Model file for the job. Use its own axes, mm. A direction names the side the tool comes from. Give positions to 0.01 mm unless a question says otherwise; leave off trailing zeros. Order: outer loops, then holes, each group sorted by start corner. A loop starts at its lowest first (then second) coordinate and runs counter-clockwise, first axis right, second up. Notation, with made-up numbers: (15.25, 45.5) -> (36.25, 45.5) arc R19 ccw to (36.25, 72.5) -> close; hole circle Ø8 at (64.5, -15.5). An arc over 180 degrees is marked (long way). Use CSV: the item, a comma, the result in double quotes. Start each with the question number.
1. Pull direction Y, two halves, no side cores. Call faces 4 (the flat face through (59, 0, 49)), 5 (the flat face through (61, 77, 49)), 6 (the flat face through (0, 79, 50)), 7 (the flat face through (61, 80, 49)): released by +Y, released by -Y, zero draft, split by the parting line, or undercut.
2. Cut at C-C on z = 71.5. List the corners of the cut face in (x, y), then the cut area to 3 significant figures.
3. Cut at D-D on z = 23. List the corners of the cut face in (x, y), then the cut area to 3 significant figures.
4. Drop flat-ended pins along their axis: pin 1 (4 mm diameter, centred on x = 115, z = 23, fed in from -Y); pin 2 (4.5 mm diameter, centred on x = 97.577, y = 59.65, fed in from -Z). Give the stop position or say it passes through.
5. Cut at A-A on x = 5. List the corners of the cut face in (y, z), then the cut area to 3 significant figures.
6. Cut at B-B on y = 20.35. List the corners of the cut face in (x, z), then the cut area to 3 significant figures.
7. 3-axis set-ups, long thin cutter, end or side, ignore diameter. For faces 1 (the cylindrical face through (39.04, 35.67, 1.52)), 2 (the flat face through (61, 41, 97)), 3 (the cylindrical face through (45.586, 19.392, 1.521)): which of +Z, -Z, +X, -X, +Y, -Y reach the whole face in a straight line?
8. Wall check: line 1 (Z direction, x = 59.5, y = 34); line 2 (Y direction, x = 107, z = 15); line 3 (Y direction, x = 40, z = 2.2) (3 decimals). Give the ranges that are in metal, low to high. Write a range as from..to.
Autodesk Inventor part; units mm, degrees
ref_plane "Work Plane1" through (0, 0, 50) normal (0, 0, 1) x (1, 0, 0)
ref_plane "YZ Plane" through (0, 0, 0) normal (1, 0, 0) x (0, 1, 0)
ref_plane "XZ Plane" through (0, 0, 0) normal (0, 1, 0) x (-1, 0, 0)
sketch "Sketch6" plane through (0, 0, 0) normal (0, 0, 1) x (1, 0, 0)
  line L0 (0, 0) -> (120, 0)
  line L1 (120, 0) -> (120, 80)
  line L2 (120, 80) -> (0, 80)
  line L3 (0, 80) -> (0, 0)
  dimension "d18" = 80
  dimension "d19" = 120
extrude "Extrusion4" add sketch "Sketch6" along normal blind 100
sketch "Sketch7" plane through (120, 0, 0) normal (1, 0, 0) x (0, 0, -1)
  line L0 (0, 0) -> (0, 80)
  line L1 (0, 80) -> (-100, 80)
  line L2 (-100, 0) -> (-100, 80)
  line L3 (0, 0) -> (-100, 0)
  line L4 (-97, 3) -> (-3, 3)
  line L5 (-3, 3) -> (-3, 77)
  line L6 (-3, 77) -> (-97, 77)
  line L7 (-97, 77) -> (-97, 3)
  point P0 (0, 0)
  dimension "d22" = 3
  dimension "d23" = 3
  dimension "d24" = 3
  dimension "d25" = 3
extrude "Extrusion5" cut sketch "Sketch7" against normal up to next contours L7 L6 L5 L4
sketch "Sketch8" plane through (0, 0, 0) normal (0, -1, 0) x (1, 0, 0)
  line L0 (0, 0) -> (120, 0)
  line L1 (120, 0) -> (120, 100)
  line L2 (0, 100) -> (120, 100)
  line L3 (0, 0) -> (0, 100)
  line L4 (120, 3) -> (0, 3)
  circle A0 centre (5, 23) radius 2.5
  circle A1 centre (115, 23) radius 2.5
  dimension "d28" = 5
  dimension "d29" = 5
  dimension "d30" = 20
  dimension "d31" = 5
  dimension "d32" = 5
  dimension "d33" = 20
extrude "Extrusion6" cut sketch "Sketch8" against normal blind 100 contours A0 | A1
sketch "Sketch9" plane through (0, 0, 100) normal (0, 0, 1) x (1, 0, 0)
  line L0 (0, 0) -> (120, 0)
  line L1 (120, 0) -> (120, 80)
  line L2 (120, 80) -> (0, 80)
  line L3 (0, 80) -> (0, 0)
  line L4 (120, 77) -> (0, 77)
  line L5 (120, 3) -> (0, 3)
  circle A0 centre (40, 40) radius 4.435
  dimension "d36" = 8.87
  dimension "d37" = 40
  dimension "d38" = 40
extrude "Extrusion7" cut sketch "Sketch9" against normal through all contours A0
ref_plane "Work Plane1" through (0, 0, 50) normal (0, 0, 1) x (1, 0, 0)
sketch "Sketch10" plane through (120, 3, 3) normal (0, 0, 1) x (1, 0, 0)
  circle A0 centre (-80, 37) radius 4.435
  line L0 (-120, 0) -> (-120, 74)
  line L1 (0, 0) -> (-120, 0)
  line L2 (0, 74) -> (0, 0)
  line L3 (0, 74) -> (-120, 74)
  circle A1 centre (-22.423, 56.65) radius 2.5
  circle A2 centre (-76.723, 17.35) radius 2.5
  line L4 (-49.573, 47.4472) -> (-49.573, 24.6677)
  point P0 (-120, -3)
  dimension "d46" = 5
  dimension "d48" = 5
  dimension "d55" = 17.35
  dimension "d58" = 30.427
  dimension "d59" = 27.15
  dimension "d72" = 17.35
  dimension "d73" = 27.15
extrude "Extrusion9" cut sketch "Sketch10" against normal blind 100 contours A1 | A2
properties part number "EE_Base-SquareBar-Rev3"
Verdict:
1,face 4,"released by -Y"
1,face 5,"undercut"
1,face 6,"zero draft"
1,face 7,"released by +Y"
2,outline,"(0, 0) -> (120, 0) -> (120, 3) -> (0, 3) -> close; (0, 77) -> (120, 77) -> (120, 80) -> (0, 80) -> close"
2,area,"720 mm^2"
3,outline,"(0, 0) -> (2.5, 0) -> (2.5, 3) -> (0, 3) -> close; (0, 77) -> (2.5, 77) -> (2.5, 80) -> (0, 80) -> close; (7.5, 0) -> (112.5, 0) -> (112.5, 3) -> (7.5, 3) -> close; (7.5, 77) -> (112.5, 77) -> (112.5, 80) -> (7.5, 80) -> close; (117.5, 0) -> (120, 0) -> (120, 3) -> (117.5, 3) -> close; (117.5, 77) -> (120, 77) -> (120, 80) -> (117.5, 80) -> close"
3,area,"660 mm^2"
4,pin 1,"through"
4,pin 2,"z = 97"
5,outline,"(0, 0) -> (80, 0) -> (80, 20.5) -> (77, 20.5) -> (77, 3) -> (3, 3) -> (3, 20.5) -> (0, 20.5) -> close; (0, 25.5) -> (3, 25.5) -> (3, 97) -> (77, 97) -> (77, 25.5) -> (80, 25.5) -> (80, 100) -> (0, 100) -> close"
5,area,"1,010 mm^2"
6,outline,"(0, 0) -> (40.78, 0) -> (40.78, 3) -> (0, 3) -> close; (0, 97) -> (120, 97) -> (120, 100) -> (0, 100) -> close; (45.78, 0) -> (120, 0) -> (120, 3) -> (45.78, 3) -> close"
6,area,"705 mm^2"
7,face 1,"+Z, -Z"
7,face 2,"+X, -X"
7,face 3,"-Z"
8,line 1,"0..3, 97..100"
8,line 2,"0..3, 77..80"
8,line 3,"0..35.565, 44.435..80"
